Could you check a few things on this drawing? It's one solid part, dimensions in mm from its lowest x, y, z. Give positions to 0.01 mm unless a question says otherwise; leave off trailing zeros. Loops run counter-clockwise (first coordinate to the right, second up) from the corner with the lowest first, then second, coordinate; pieces in that order, holes last. Notation, with made-up numbers: (-19.75, 74.5) - (25.25, 74.5) arc R18 ccw to (25.25, 87.5) - close; hole circle Ø8 at (-35, 29.5). An arc over 180 degrees is marked (long way). Return JSON: item names as keys, results as strings. Group by question number.
(1) If we section it at A-A (z = 15): Please give me the cut outline in (x, y), then the cut area to 3 significant figures.
(2) If we section it at B-B (x = 73.2): Please give me the cut outline in (y, z), then the cut area to 4 significant figures.
(3) I need wall thicknesses on probe 1 along X at (y, z) = (3.95, 15); probe 2 along Z at (x, y) = (73.2, 2.9). Which ranges of each line are inside material? Lowest first, please. Write a range as [from, to].
(4) For P1, Ø3.5, axis at x = 73.2, z = 201, coming from the +Y side, with a flat end and sliding along its axis, tell me the tip position at first contact or that it passes through.
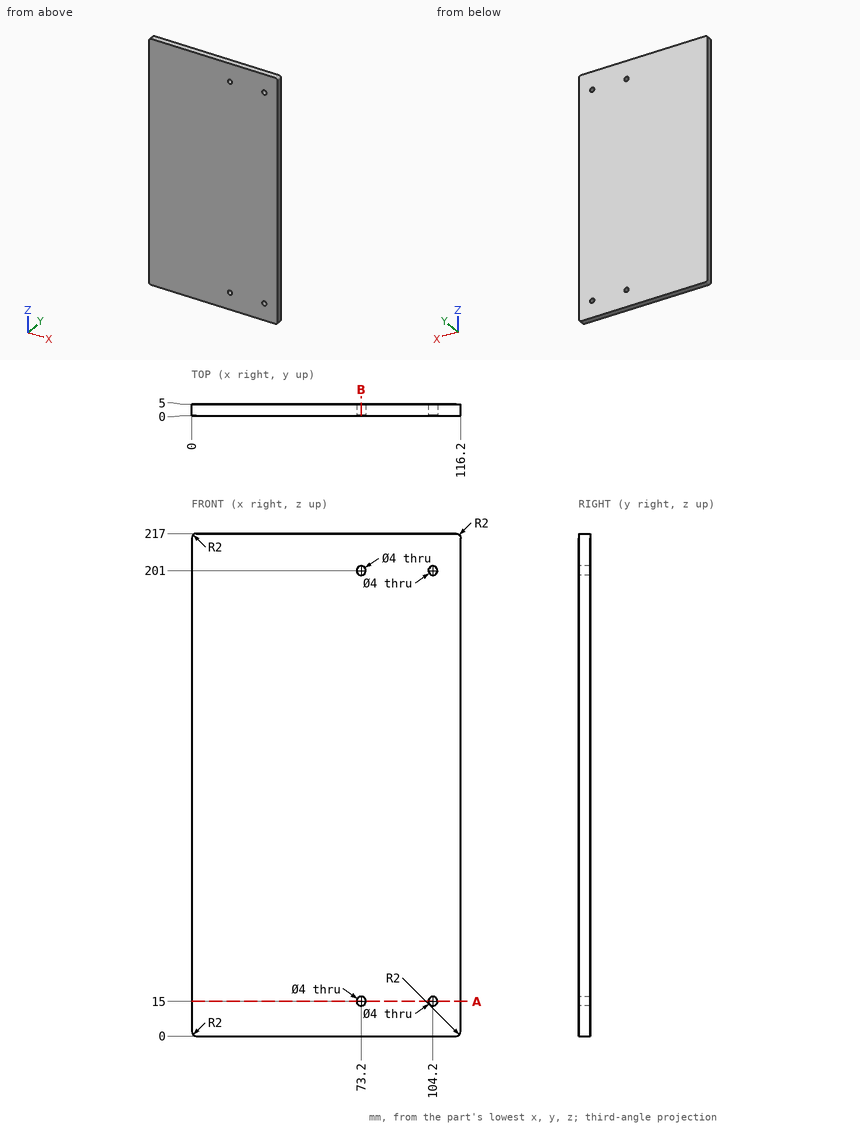
Values:
{
 "1": {"outline": "(0, 0) - (71.2, 0) - (71.2, 5) - (0, 5) - close; (75.2, 0) - (102.2, 0) - (102.2, 5) - (75.2, 5) - close; (106.2, 0) - (116.2, 0) - (116.2, 5) - (106.2, 5) - close", "area": "541 mm2"},
 "2": {"outline": "(0, 0) - (5, 0) - (5, 13) - (0, 13) - close; (0, 17) - (5, 17) - (5, 199) - (0, 199) - close; (0, 203) - (5, 203) - (5, 217) - (0, 217) - close", "area": "1,045 mm2"},
 "3": {"probe 1": "[0, 71.2], [75.2, 102.2], [106.2, 116.2]", "probe 2": "[0, 13], [17, 199], [203, 217]"},
 "4": {"P1": "through"}
}
